```python
from build123d import *

# Parameters (mm, degrees)
F0_W     = 16.9495176524
F0_H     = 58.9220710099
F1_DEPTH = 18.034
F2_DEPTH = 71.12
F3_R     = 5.08
F4_R     = 5.367457486
F5_DEPTH = 30.226


with BuildPart() as f1:
    # F0 (on Front) → F1 (new body)
    with BuildSketch(Plane.XZ):
        with Locations((-8.4747588262, 29.4610355049)):
            Rectangle(F0_W, F0_H)
    extrude(amount=F1_DEPTH)

    # F2 (add): a face of the model
    f2_faces = [f1.faces().sort_by_distance(p)[0] for p in [
        (-8.4747588262, -9.017, 58.9220710099),
    ]]
    extrude(f2_faces, amount=F2_DEPTH)

    # F3
    f3_edges = [f1.edges().sort_by_distance(p)[0] for p in [
        (-8.474759, -18.034, 130.042071),
        (0, -9.017, 130.042071),
        (-8.474759, 0, 130.042071),
        (-16.949518, -9.017, 130.042071),
    ]]
    fillet(f3_edges, radius=F3_R)

    # F4 (on face) → F5 (join)
    with BuildSketch(Plane.YZ):
        with Locations((-9.8099326715, 110.4333996773)):
            Circle(F4_R)
    extrude(amount=F5_DEPTH)


solid = f1.part
```
For this review, take the finished solid that the model builds, in its own axes (mm). A direction names the side the tool comes from. Coordinates: 2 decimals unless noted, no trailing zeros. Write each loop counter-clockwise with the first axis right and the second up, starting at its lowest first coordinate (ties: lowest second). Pieces come first, ordered by that corner, then holes. Notation, with made-up numbers: (-37, -3) -> (-5, -3) arc R7 ccw to (-5, 4) -> close; hole circle Ø7 at (46.5, 14). An arc over 180 degrees is marked (long way). Put each result on its own line as item: value.
Q1. Take a section at C-C, the plane x = 1.5. State the section outline as (y, z) points, then the cut area to 3 significant figures.
From the geometry:
outline: circle Ø10.73 at (-9.81, 110.43)
area: 90.5 mm2
Q2. Take a section at B-B, the plane z = 17. State the section outline as (x, y) points.
From the geometry:
outline: (-16.95, -18.03) -> (0, -18.03) -> (0, 0) -> (-16.95, 0) -> close
Q3. Tool access review of faces 1 (the cylindrical face through (-0.887, -9.143, 127.83)), 2 (the cylindrical face through (14.901, -10.509, 115.755)): name each direction out of +Z, -Z, +X, -X, +Y, -Y from which nothing blocks a thin tool from reaching the whole face with its end or side.
From the geometry:
face 1: +Z, +X, +Y, -Y
face 2: +X
Q4. Take a section at A-A, the plane y = -3. State the section outline as (x, z) points, then the cut area to 3 significant figures.
From the geometry:
outline: (-16.95, 0) -> (0, 0) -> (0, 124.96) arc R5.08 ccw to (-3, 129.6) -> (-13.95, 129.6) arc R5.08 ccw to (-16.95, 124.96) -> close
area: 2,190 mm2
Q5. Clearance check with flat-ended pins moving along their axes: pin 1 Ø5 at (x, y) = (13, -3) entering from +Z; pin 2 Ø8 at (x, y) = (1.5, -3) entering from -Z; pin 3 Ø3 at (x, y) = (15, -8.5) entering from -Z. State where each tip first meets the part, or that it passes through.
From the geometry:
pin 1: stops at z = 113.63
pin 2: stops at z = 0
pin 3: stops at z = 105.07
Q6. Wall thickness on L1, parallel to X at y = -10, z = 17.5; L2, parallel to Z at x = 4, y = -10; L3, parallel to Z at x = 22, y = -5: over which ranges is each line inside the solid? List them lowest first.
From the geometry:
L1: x = -16.95 to 0
L2: z = 105.07 to 115.8
L3: z = 108.05 to 112.82
